```python
from build123d import *

# Parameters (mm, degrees)
SKETCH2_R           = 2
BOSS_EXTRUDE1_DEPTH = 10
FILLET2_R           = 3


with BuildPart() as part:
    # Sketch2 → Boss-Extrude1 (new body)
    with BuildSketch(Plane.XY):
        with BuildLine():
            Line((8, 50), (8, -50))
            ThreePointArc((8, -50), (0, -58), (-8, -50))
            Line((-8, -50), (-8, 50))
            ThreePointArc((-8, 50), (0, 58), (8, 50))
        make_face()
        with Locations((0, 50)):
            Circle(SKETCH2_R, mode=Mode.SUBTRACT)
        with Locations((0, -50)):
            Circle(SKETCH2_R, mode=Mode.SUBTRACT)
    extrude(amount=BOSS_EXTRUDE1_DEPTH)

    # Fillet2
    fillet2_edges = [part.edges().sort_by_distance(p)[0] for p in [
        (0, -58, 10),
        (8, 0, 10),
        (0, 58, 10),
        (8, 0, 0),
        (0, -58, 0),
        (-8, 0, 0),
        (0, 58, 0),
        (-8, 0, 10),
    ]]
    fillet(fillet2_edges, radius=FILLET2_R)


solid = part.part
```
The model under review builds one solid part; all positions refer to its coordinate system, in mm. Round coordinates to 2 decimals unless told otherwise and drop trailing zeros. Write each loop counter-clockwise with the first axis right and the second up, starting at its lowest first coordinate (ties: lowest second). Pieces come first, ordered by that corner, then holes. Notation, with made-up numbers: (87.5, 68) - (111.5, 68) arc R24 ccw to (111.5, 78) - close; hole circle Ø5 at (-4, 86). An arc over 180 degrees is marked (long way). One line per question, with ' | ' between items.
Item 1: To check wall thickness, follow probe 1 along Y at (x, z) = (0, 7); probe 2 along Y at (x, z) = (0, 8); probe 3 along X at (y, z) = (-51, 8.25). State the ranges of each line that lie inside material, in increasing order.
Resolved:
probe 1: y = -58 to -52, -48 to 48, 52 to 58 | probe 2: y = -57.83 to -52, -48 to 48, 52 to 57.83 | probe 3: x = -7.66 to -1.73, 1.73 to 7.66
Item 2: For P1, Ø1, axis at x = -4, z = 5.5, coming from the +Y side; P2, Ø5, axis at x = 3.5, z = 4.5, coming from the -Y side; P3, Ø3, axis at x = 5, z = 1.5, coming from the +Y side, all flat-tipped, find the tip position at first contact; note any pin that passes through.
Resolved:
P1: stops at y = 57.19 | P2: stops at y = -57.94 | P3: stops at y = 56.98
Item 3: Add section A-A, the plane y = -31. Give the boundary of the cut face in (x, z).
Resolved:
outline: (-8, 3) arc R3 ccw to (-5, 0) - (5, 0) arc R3 ccw to (8, 3) - (8, 7) arc R3 ccw to (5, 10) - (-5, 10) arc R3 ccw to (-8, 7) - close
Item 4: Add section B-B, the plane x = 0. Give the boundary of the cut face in (y, z), then the cut area to 3 significant figures.
Resolved:
outline: (-58, 3) arc R3 ccw to (-55, 0) - (-52, 0) - (-52, 10) - (-55, 10) arc R3 ccw to (-58, 7) - close; (-48, 0) - (48, 0) - (48, 10) - (-48, 10) - close; (52, 0) - (55, 0) arc R3 ccw to (58, 3) - (58, 7) arc R3 ccw to (55, 10) - (52, 10) - close | area: 1,070 mm2
Item 5: Add section C-C, the plane z = 1.5. Give the boundary of the cut face in (x, y).
Resolved:
outline: (-7.6, -50) arc R7.6 ccw to (7.6, -50) - (7.6, 50) arc R7.6 ccw to (-7.6, 50) - close; hole circle Ø4 at (0, -50); hole circle Ø4 at (0, 50)
Item 6: The part is to be moulded in two halves that separate along X. For faces 1 (the face through (7.14, -0.7, 0.9)), 2 (the face through (0, 58, 5)), 3 (the face through (0.923, 48.226, 4.93)), 4 (the face through (0.923, -51.774, 4.93)), say which applies: pulls with the +X half, pulls with the -X half, needs draft (parallel to the pull), parting line crosses it, or undercut.
Resolved:
face 1: pulls with the +X half | face 2: parting line crosses it | face 3: undercut | face 4: undercut
